Design review of the part built by this model. Coordinates are the model's own, in mm. Coordinates: 2 decimals unless noted, no trailing zeros. Write each loop counter-clockwise with the first axis right and the second up, starting at its lowest first coordinate (ties: lowest second). Pieces come first, ordered by that corner, then holes. Notation, with made-up numbers: M 36.25,86.25 L 84.25,86.25 A11 cw 84.25,96.25 Z; hole C 0,15.5 d2. An arc over 180 degrees is marked long. One line per question, with ' | ' between items.
Autodesk Inventor part; units mm, degrees
ref_plane "YZ Plane" through (0, 0, 0) normal (1, 0, 0) x (0, 1, 0)
ref_plane "XZ Plane" through (0, 0, 0) normal (0, 1, 0) x (-1, 0, 0)
ref_plane "XY Plane" through (0, 0, 0) normal (0, 0, 1) x (1, 0, 0)
sketch "Skizze1" plane through (0, 0, 0) normal (0, 1, 0) x (-1, 0, 0)
  line L0 (0, 0) -> (25, 0)
  line L1 (25, 0) -> (25, -22)
  line L2 (25, -22) -> (0, -22)
  line L3 (0, -22) -> (0, 0)
  dimension "d0" = 25
  dimension "d1" = 22
extrude "Extrusion1" add sketch "Skizze1" along normal blind 2
chamfer "Fase1" distance 9 angle 45 4 edges at (0, 1, 0) (0, 1, -22) (-25, 1, -22) (-25, 1, 0)
fillet "Rundung1" radius 4 8 edges at (-25, 1, -13) (-25, 1, -9) (-16, 1, 0) (-9, 1, 0) (0, 1, -9) (0, 1, -13) (-9, 1, -22) (-16, 1, -22)
sketch "Skizze2" plane through (0, 2, 0) normal (0, 1, 0) x (1, 0, 0)
  line L0 (0, 10.6569) -> (0, 11.3431)
  line L1 (-14.3431, 0) -> (-10.6569, 0)
  point P0 (0, 0)
  point P1 (-2.25, 11)
  point P2 (-22.75, 11)
  dimension "d8" = 2.25
  dimension "d9" = 20.5
  dimension "d10" = 11
sketch "Skizze3" plane through (0, 2, 0) normal (0, 1, 0) x (1, 0, 0)
  line L0 (-14.3431, 0) -> (-10.6569, 0)
  line L1 (0, 10.6569) -> (0, 11.3431)
  point P0 (0, 0)
  point P1 (-12.5, 3)
  point P2 (-12.5, 19)
  dimension "d11" = 16
  dimension "d12" = 3
  dimension "d13" = 12.5
hole "Bohrung1" at (-12.5, 2, -3) at (-12.5, 2, -19) direction (0, -1, 0) diameter 3 depth 8 tip angle 118
hole "Bohrung2" at (-2.25, 2, -11) at (-22.75, 2, -11) direction (0, -1, 0) diameter 3 depth 8 tip angle 118
properties part number "KugelradAdapter"
1. Take a section at B-B (x = -22.75). Write out the cut boundary in (y, z).
Answer sheet:
outline: M 0,-15.25 L 2,-15.25 L 2,-12.5 L 0,-12.5 Z; M 0,-9.5 L 2,-9.5 L 2,-6.75 L 0,-6.75 Z
2. Insertion check: pin 1 Ø1.5 at (x, z) = (-5, -16) entering from -Y; pin 2 Ø2.5 at (x, z) = (-12.5, -19) entering from +Y. Each pin has a flat end and moves straight along its axis. Give the tip position at first contact, or say it passes through.
Answer sheet:
pin 1: y = 0 | pin 2: through
3. Draft analysis for pull direction X (two halves, no side actions). For faces 1 (the face through (-12, 1, 0)), 2 (the face through (-21, 1, -5)), 3 (the face through (-24.237, 0.986, -11.195)), state which applies: pulls with the +X half, pulls with the -X half, needs draft (parallel to the pull), parting line crosses it, or undercut.
Answer sheet:
face 1: needs draft | face 2: pulls with the -X half | face 3: undercut
4. To check wall thickness, follow line 1 along Z through (x, y) = (-12.5, 1.1); line 2 along Z through (x, y) = (-13.25, 0.2); line 3 along X through (y, z) = (0.8, -12.25). State the ranges of each line that lie inside material, in increasing order. Write a range as [from, to].
Answer sheet:
line 1: [-22, -20.5], [-17.5, -4.5], [-1.5, 0] | line 2: [-22, -20.3], [-17.7, -4.3], [-1.7, 0] | line 3: [-24.9, -23.58], [-21.92, -3.08], [-1.42, -0.1]
5. Take a section at D-D (z = -11). Write out the cut boundary in (x, y).
Answer sheet:
outline: M -25,0 L -24.25,0 L -24.25,2 L -25,2 Z; M -21.25,0 L -3.75,0 L -3.75,2 L -21.25,2 Z; M -0.75,0 L 0,0 L 0,2 L -0.75,2 Z
6. Take a section at C-C (y = 1.3). Write out the cut boundary in (x, z).
Answer sheet:
outline: M -25,-11.34 A4 ccw -23.83,-14.17 L -17.17,-20.83 A4 ccw -14.34,-22 L -10.66,-22 A4 ccw -7.83,-20.83 L -1.17,-14.17 A4 ccw 0,-11.34 L 0,-10.66 A4 ccw -1.17,-7.83 L -7.83,-1.17 A4 ccw -10.66,0 L -14.34,0 A4 ccw -17.17,-1.17 L -23.83,-7.83 A4 ccw -25,-10.66 Z; hole C -22.75,-11 d3; hole C -12.5,-19 d3; hole C -12.5,-3 d3; hole C -2.25,-11 d3
7. Take a section at A-A (z = -3). Write out the cut boundary in (x, y).
Answer sheet:
outline: M -19,0 L -14,0 L -14,2 L -19,2 Z; M -11,0 L -6,0 L -6,2 L -11,2 Z
